Can you work these out from the model? Positions are in its coordinate system, mm. Round coordinates to 2 decimals unless told otherwise and drop trailing zeros. Loops run counter-clockwise (first coordinate to the right, second up) from the corner with the lowest first, then second, coordinate; pieces in that order, holes last. Notation, with made-up numbers: (59.5, 83.25) -> (72.5, 83.25) arc R31 ccw to (72.5, 119.25) -> close; hole circle Ø11 at (-17.75, 77.5). An arc over 180 degrees is marked (long way). Use a Markdown table: item, result.
from build123d import *

# Parameters (mm, degrees)
BOSS_EXTRUDE1_DEPTH   = 15
M6_TAPPED_HOLE1_D     = 5
M6_TAPPED_HOLE1_DEPTH = 10
M6_TAPPED_HOLE1_TIP   = 1.502151548
M6_TAPPED_HOLE2_D     = 5
M6_TAPPED_HOLE2_DEPTH = 10
M6_TAPPED_HOLE2_TIP   = 1.502151548


with BuildPart() as part:
    # Sketch1 → Boss-Extrude1 (new body)
    with BuildSketch(Plane(origin=(0, 0, 0), x_dir=(1, 0, 0), z_dir=(0, 1, 0))):
        Polygon((0, 0), (0, -125), (-20, -125), (-45, -20), (-45, 0), align=None)
    extrude(amount=BOSS_EXTRUDE1_DEPTH)

    # M6 Tapped Hole1
    with Locations(Plane(origin=(0, 0, 0), x_dir=(-1, 0, 0), z_dir=(0, 0, -1))):
        with Locations((35, 7.5)):
            Hole(M6_TAPPED_HOLE1_D / 2, depth=M6_TAPPED_HOLE1_DEPTH)
            with Locations((0, 0, -(M6_TAPPED_HOLE1_DEPTH + M6_TAPPED_HOLE1_TIP / 2))):  # 118° drill point
                Cone(0, M6_TAPPED_HOLE1_D / 2, M6_TAPPED_HOLE1_TIP, mode=Mode.SUBTRACT)

    # M6 Tapped Hole2
    with Locations(Plane(origin=(0, 0, 0), x_dir=(0, 0, -1), z_dir=(1, 0, 0))):
        with Locations((-105, 7.5), (-62.5, 7.5), (-20, 7.5)):
            Hole(M6_TAPPED_HOLE2_D / 2, depth=M6_TAPPED_HOLE2_DEPTH)
            with Locations((0, 0, -(M6_TAPPED_HOLE2_DEPTH + M6_TAPPED_HOLE2_TIP / 2))):  # 118° drill point
                Cone(0, M6_TAPPED_HOLE2_D / 2, M6_TAPPED_HOLE2_TIP, mode=Mode.SUBTRACT)


solid = part.part
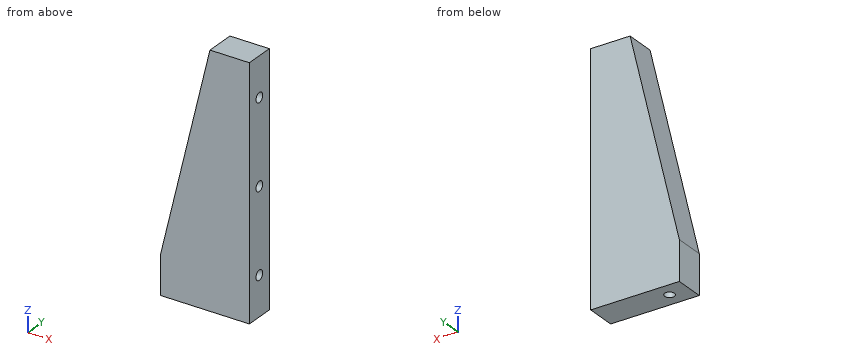
1. I need wall thicknesses on line 1 (Z direction, x = -4.5, y = 7.5); line 2 (Y direction, x = -3.5, z = 20); line 3 (X direction, y = 7.5, z = 4.5). Which ranges of each line are inside material? Lowest first, please.
Answer sheet:
| item | result |
|---|---|
| line 1 | z = 0 to 17.5, 22.5 to 60, 65 to 102.5, 107.5 to 125 |
| line 2 | y = 0 to 5, 10 to 15 |
| line 3 | x = -45 to -37.5, -32.5 to 0 |
2. I want a section at D-D (z = 96.5). Please give me the cut outline in (x, y).
Answer sheet:
| item | result |
|---|---|
| outline | (-26.79, 0) -> (0, 0) -> (0, 15) -> (-26.79, 15) -> close |
3. Will these pins go through, and if not, where does the flat tip stop? pin 1 Ø1.5 at (y, z) = (10, 57.5) entering from +X; pin 2 Ø4 at (y, z) = (7.5, 62.5) entering from -X; pin 3 Ø6 at (y, z) = (7.5, 105) entering from -X.
Answer sheet:
| item | result |
|---|---|
| pin 1 | stops at x = 0 |
| pin 2 | stops at x = -35.36 |
| pin 3 | stops at x = -25.48 |
4. I want a section at B-B (y = 3). Please give me the cut outline in (x, z), plus the area to 3 significant figures.
Answer sheet:
| item | result |
|---|---|
| outline | (-45, 0) -> (0, 0) -> (0, 125) -> (-20, 125) -> (-45, 20) -> close |
| area | 4,310 mm² |
5. I want a section at C-C (x = -41). Please give me the cut outline in (y, z).
Answer sheet:
| item | result |
|---|---|
| outline | (0, 0) -> (15, 0) -> (15, 36.8) -> (0, 36.8) -> close |
6. I want a section at A-A (x = -4). Please give me the cut outline in (y, z).
Answer sheet:
| item | result |
|---|---|
| outline | (0, 0) -> (15, 0) -> (15, 125) -> (0, 125) -> close; hole circle Ø5 at (7.5, 20); hole circle Ø5 at (7.5, 62.5); hole circle Ø5 at (7.5, 105) |
